from build123d import *

# Parameters (mm, degrees)
SKETCH_W        = 45
SKETCH_H        = 70
SKETCH_R        = 2.25
PAD_DEPTH       = 15
SKETCH001_R     = 10.6
POCKET_DEPTH    = 70.001
SKETCH002_R     = 4.6
POCKET001_DEPTH = 4


with BuildPart() as part:
    # Sketch → Pad (new body)
    with BuildSketch(Plane.XY):
        Rectangle(SKETCH_W, SKETCH_H)
        with Locations((-16.7, 30)):
            Circle(SKETCH_R, mode=Mode.SUBTRACT)
        with Locations((16.7, 30)):
            Circle(SKETCH_R, mode=Mode.SUBTRACT)
        with Locations((-16.7, -30)):
            Circle(SKETCH_R, mode=Mode.SUBTRACT)
        with Locations((16.7, -30)):
            Circle(SKETCH_R, mode=Mode.SUBTRACT)
        with Locations((-16.7, 0)):
            Circle(SKETCH_R, mode=Mode.SUBTRACT)
        with Locations((16.7, 0)):
            Circle(SKETCH_R, mode=Mode.SUBTRACT)
        with Locations((16.7, 15)):
            Circle(SKETCH_R, mode=Mode.SUBTRACT)
        with Locations((-16.7, 15)):
            Circle(SKETCH_R, mode=Mode.SUBTRACT)
    extrude(amount=PAD_DEPTH)

    # Sketch001 → Pocket (cut, through all)
    with BuildSketch(Plane.XZ.offset(35)):
        with Locations((0, 15)):
            Circle(SKETCH001_R)
    extrude(amount=-POCKET_DEPTH, mode=Mode.SUBTRACT)

    # Sketch002 → Pocket001 (cut)
    with BuildSketch(Plane.XY.offset(15)):
        with Locations((-16.7, 15)):
            Circle(SKETCH002_R)
        with Locations((16.7, 15)):
            Circle(SKETCH002_R)
    extrude(amount=-POCKET001_DEPTH, mode=Mode.SUBTRACT)


solid = part.part
Read the model definition and answer for the solid it produces. Units are mm, in the model's axes. A direction names the side the tool comes from. Coordinates: 2 decimals unless noted, no trailing zeros. Loops run counter-clockwise (first coordinate to the right, second up) from the corner with the lowest first, then second, coordinate; pieces in that order, holes last.
Q1. The mould has two halves that part along X. Classify faces 3 (the face through (-18.486, -31.369, 7.395)), 4 (the face through (22.5, 0, 7)), 5 (the face through (0, -35, 4)): +X half, -X half, draft (parallel to the pull), parting line (faces both ways), or undercut.
Q2. Each of these flat-tipped pins is pushed along its axis until it touches: pin 1 Ø3 at (x, y) = (7.5, 21) entering from -Z; pin 2 Ø3.5 at (x, y) = (16.7, 15) entering from -Z; pin 3 Ø7.5 at (x, y) = (-16.7, 15) entering from +Z. Where does it stop, or does it pass through?
Q3. Consider probe 1 along Y at (x, z) = (16.7, 11.5); probe 2 along Y at (x, z) = (-16.7, 4.5); probe 3 along X at (y, z) = (-28.5, 3.25). Determine where each line is inside the solid, lowest interval first.
Q4. The part is cut by section D-D on x = 16.5. Write down the section's boundary in (y, z).
Q5. The part is cut by section A-A on y = 15. Write down the section's boundary in (x, z), and give its area (3 significant figures).
Q6. The part is cut by section B-B on x = -16.7. Write down the section's boundary in (y, z), and give its area (3 significant figures).
Q7. The part is cut by section C-C on y = 0. Write down the section's boundary in (x, z).
Q8. Which of the six approach directions +Z, -Z, +X, -X, +Y, -Y give full straight-line access (tool end or side, diameter ignored) to faces 1 (the face through (0, 35, 4)), 2 (the face through (21.09, 16.38, 13.03))?
Results below:
1. face 3: undercut
1. face 4: +X half
1. face 5: draft
2. pin 1: stops at z = 0
2. pin 2: passes through
2. pin 3: stops at z = 11
3. probe 1: y = -35 to -32.25, -27.75 to -2.25, 2.25 to 10.4, 19.6 to 27.75, 32.25 to 35
3. probe 2: y = -35 to -32.25, -27.75 to -2.25, 2.25 to 12.75, 17.25 to 27.75, 32.25 to 35
3. probe 3: x = -22.5 to -18.38, -15.02 to 15.02, 18.38 to 22.5
4. outline: (-35, 0) - (-32.24, 0) - (-32.24, 15) - (-35, 15) - close; (-27.76, 0) - (-2.24, 0) - (-2.24, 15) - (-27.76, 15) - close; (2.24, 0) - (12.76, 0) - (12.76, 11) - (10.4, 11) - (10.4, 15) - (2.24, 15) - close; (17.24, 0) - (27.76, 0) - (27.76, 15) - (19.6, 15) - (19.6, 11) - (17.24, 11) - close; (32.24, 0) - (35, 0) - (35, 15) - (32.24, 15) - close
5. outline: (-22.5, 0) - (-18.95, 0) - (-18.95, 11) - (-21.3, 11) - (-21.3, 15) - (-22.5, 15) - close; (-14.45, 0) - (14.45, 0) - (14.45, 11) - (12.1, 11) - (12.1, 15) - (10.6, 15) arc R10.6 cw to (-10.6, 15) - (-12.1, 15) - (-12.1, 11) - (-14.45, 11) - close; (18.95, 0) - (22.5, 0) - (22.5, 15) - (21.3, 15) - (21.3, 11) - (18.95, 11) - close
5. area: 326 mm2
6. outline: (-35, 0) - (-32.25, 0) - (-32.25, 15) - (-35, 15) - close; (-27.75, 0) - (-2.25, 0) - (-2.25, 15) - (-27.75, 15) - close; (2.25, 0) - (12.75, 0) - (12.75, 11) - (10.4, 11) - (10.4, 15) - (2.25, 15) - close; (17.25, 0) - (27.75, 0) - (27.75, 15) - (19.6, 15) - (19.6, 11) - (17.25, 11) - close; (32.25, 0) - (35, 0) - (35, 15) - (32.25, 15) - close
6. area: 761 mm2
7. outline: (-22.5, 0) - (-18.95, 0) - (-18.95, 15) - (-22.5, 15) - close; (-14.45, 0) - (14.45, 0) - (14.45, 15) - (10.6, 15) arc R10.6 cw to (-10.6, 15) - (-14.45, 15) - close; (18.95, 0) - (22.5, 0) - (22.5, 15) - (18.95, 15) - close
8. face 1: +Z, -Z, +X, -X, +Y
8. face 2: +Z
